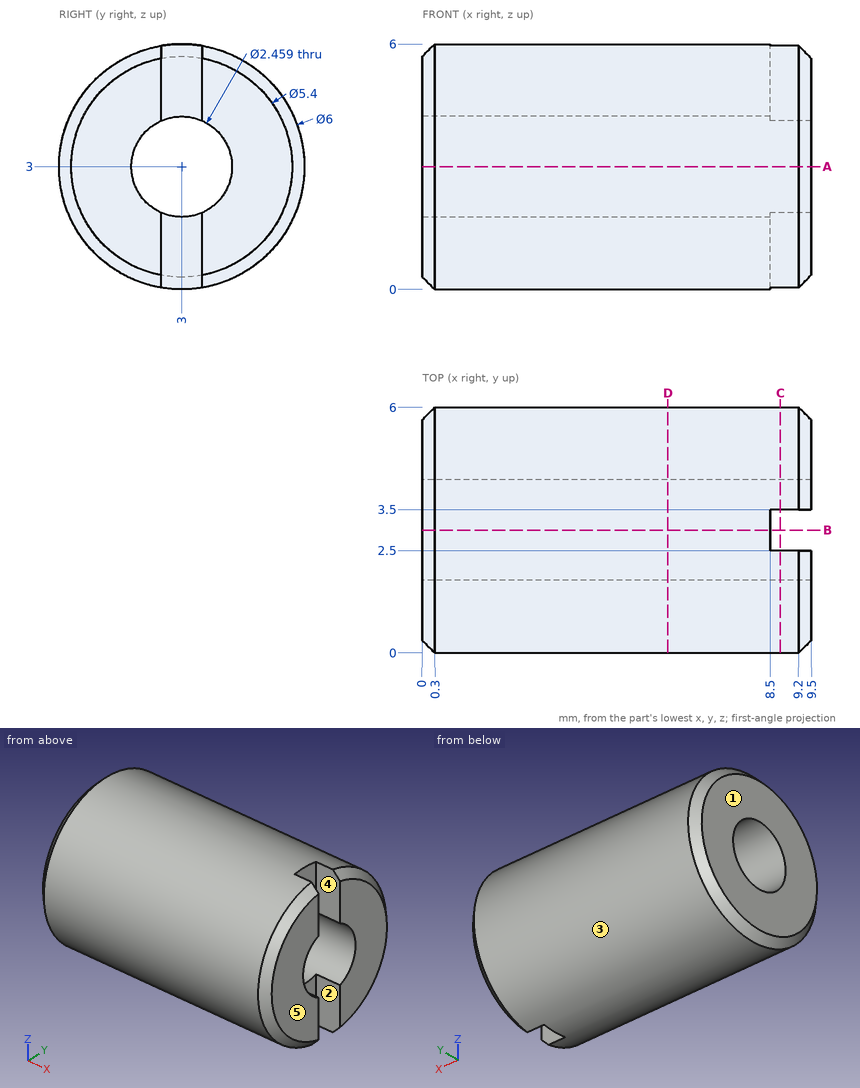
Geometry: see drawing. Coordinates: mm, zero at the bounding-box minimum. A direction names the side the tool comes from. Give positions to 0.01 mm unless a question says otherwise; leave off trailing zeros. Write each loop counter-clockwise with the first axis right and the second up, starting at its lowest first coordinate (ties: lowest second). Pieces come first, ordered by that corner, then holes. Notation, with made-up numbers: (62.5, 31) - (73.5, 31) arc R22 ccw to (73.5, 50) - close; hole circle Ø11 at (80.25, -7.5). An arc over 180 degrees is marked (long way). Return JSON: item names as keys, results as strings. Group by question number.
1) Section D-D on x = 6. Return the cut outline in (y, z).
2) Section A-A on z = 3. Return the cut outline in (x, y).
3) Mould query, pull axis Y, two halves, no side actions, for the marked faces 1, 2 and 3. Classes: released by +Y, released by -Y, zero draft, split by the parting line, or undercut.
4) Line query: line 1 (Y direction, x = 4.75, z = 3); line 2 (Y direction, x = 8, z = 2.5); line 3 (Z direction, x = 1.5, y = 1). Output: solid intervals per line, ascending.
5) Section B-B on y = 3. Return the cut outline in (x, z), plus the area to 3 significant figures.
6) First-contact query: P1, Ø0.5, axis at x = 9, z = 1, coming from the +Y side; P2, Ø1.1, axis at x = 9, z = 5, coming from the -Y side; P3, Ø0.8, axis at x = 9, z = 1.5, coming from the -Y side. Flat tips, straight axial feed; report the tip coordinate or a pass-through.
7) Set-up query: the marked faces 4 and 5. Return all of +Z, -Z, +X, -X, +Y, -Y with unobstructed straight access to the full face (end or side cutting, diameter ignored); none if empty.
8) Section C-C on x = 8.75. Return the cut outline in (y, z), plus the area to 3 significant figures.
Filled in:
{
 "1": {"outline": "circle Ø6 at (3, 3); hole circle Ø2.46 at (3, 3)"},
 "2": {"outline": "(0, 0.3) - (0.3, 0) - (9.2, 0) - (9.5, 0.3) - (9.5, 1.77) - (0, 1.77) - close; (0, 4.23) - (9.5, 4.23) - (9.5, 5.7) - (9.2, 6) - (0.3, 6) - (0, 5.7) - close"},
 "3": {"face 1": "zero draft", "face 2": "undercut", "face 3": "split by the parting line"},
 "4": {"line 1": "y = 0 to 1.77, 4.23 to 6", "line 2": "y = 0.04 to 1.88, 4.12 to 5.96", "line 3": "z = 0.76 to 5.24"},
 "5": {"outline": "(0, 0.3) - (0.3, 0) - (8.5, 0) - (8.5, 1.77) - (0, 1.77) - close; (0, 4.23) - (8.5, 4.23) - (8.5, 6) - (0.3, 6) - (0, 5.7) - close", "area": "30.0 mm^2"},
 "6": {"P1": "stops at y = 5.44", "P2": "stops at y = 0.37", "P3": "stops at y = 0.21"},
 "7": {"face 4": "+Z, -Z, +X", "face 5": "+Z, -Z, +X, +Y, -Y"},
 "8": {"outline": "(2.5, 0.04) - (2.5, 1.88) arc R1.23 cw to (2.5, 4.12) - (2.5, 5.96) arc R3 ccw to start; (3.5, 0.04) arc R3 ccw to (3.5, 5.96) - (3.5, 4.12) arc R1.23 cw to (3.5, 1.88) - close", "area": "19.9 mm^2"}
}
